```python
from build123d import *

# Parameters (mm, degrees)
F1_DEPTH = 25.4


with BuildPart() as f1:
    # F0 (on Right) → F1 (new body)
    with BuildSketch(Plane.YZ):
        with BuildLine():
            Line((9.737576, 0), (0, 0))
            Line((0, 0), (0, -69.85))
            ThreePointArc((0, -69.85), (1.859872, -74.340128), (6.35, -76.2))
            Line((6.35, -76.2), (88.985146, -76.2))
            Line((88.985146, -76.2), (88.985146, -70.901472))
            Line((88.985146, -70.901472), (44.77061, -65.602944))
            Line((44.77061, -65.602944), (9.737576, -65.602944))
            Line((9.737576, -65.602944), (9.737576, 0))
        make_face()
    extrude(amount=F1_DEPTH)


solid = f1.part
```
Could you check a few things on this model? Use its own coordinates, in mm. A direction names the side the tool comes from. Round coordinates to 2 decimals unless told otherwise and drop trailing zeros. Order: outer loops, then holes, each group sorted by start corner. A loop starts at its lowest first (then second) coordinate and runs counter-clockwise, first axis right, second up. Notation, with made-up numbers: M 60,87.25 L 91,87.25 A25 cw 91,121.25 Z; hole C 52.25,34.25 d8. An arc over 180 degrees is marked long. One line per question, with ' | ' between items. Start each with the question number.
(1) Suppose I cut it at A-A on x = 6. List the corners of the cut face in (y, z) for me, then the cut area to 3 significant figures.
(2) Suppose I cut it at B-B on z = -44. List the corners of the cut face in (x, y) for me.
(3) Suppose I cut it at C-C on y = 31. List the corners of the cut face in (x, z) for me.
(4) For faces 1 (the face through (13, 9.738, -33)), 2 (the face through (13, 5, 0)), which set-ups out of +Z, -Z, +X, -X, +Y, -Y let a thin tool reach every point of the face, with its end or its side?
(5) For P1, Ø10, axis at x = 11, y = 41.5, coming from the +Z side; P2, Ø4, axis at x = 4.5, z = -14.5, coming from the +Y side, each with a flat end and sliding along its axis, tell me the tip position at first contact or that it passes through.
(6) Please list where these lines run through material, in increasing order: line 1 along Z through (x, y) = (4.25, 41); line 2 along Y through (x, z) = (17.25, -21); line 3 along Z through (x, y) = (5, 70.5).
Geometry results:
1) outline: M 0,-69.85 A6.35 ccw 6.35,-76.2 L 88.99,-76.2 L 88.99,-70.9 L 44.77,-65.6 L 9.74,-65.6 L 9.74,0 L 0,0 Z | area: 1,460 mm²
2) outline: M 0,0 L 25.4,0 L 25.4,9.74 L 0,9.74 Z
3) outline: M 0,-76.2 L 25.4,-76.2 L 25.4,-65.6 L 0,-65.6 Z
4) face 1: +Z, +X, -X, +Y | face 2: +Z, +X, -X, +Y, -Y
5) P1: z = -65.6 | P2: y = 9.74
6) line 1: -76.2 to -65.6 | line 2: 0 to 9.74 | line 3: -76.2 to -68.69
